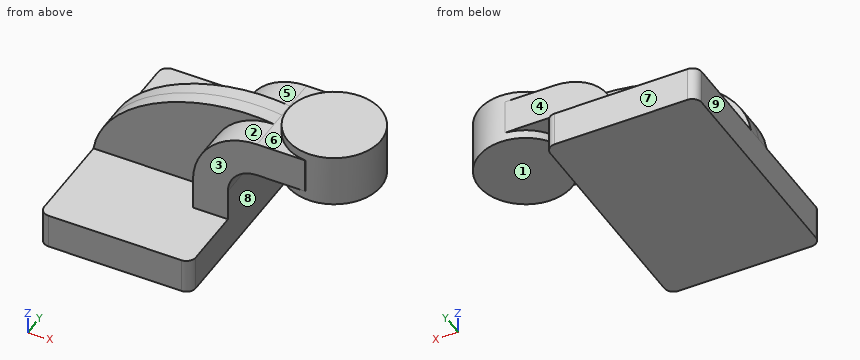
from build123d import *

# Parameters (mm, degrees)
F1_DEPTH = 63.5
F0_W     = 23.0290793641
F0_H     = 19.05
F2_DEPTH = 25.4
F3_DEPTH = 7.9375
F5_R     = 5.08


with BuildPart() as f1:
    # F0 (on Front) → F1 (new body, symmetric)
    with BuildSketch(Plane.XZ):
        Polygon((-41.275, 9.525), (-41.275, -9.525), (41.275, -9.525), (41.275, 9.525), (22.225, 9.525), align=None)
    extrude(amount=F1_DEPTH, both=True)

    # F0 (on Front) → F2 (join, symmetric)
    with BuildSketch(Plane.XZ):
        with Locations((71.839539682, 52.4002)):
            Rectangle(F0_W, F0_H)
        with BuildLine():
            Line((22.225, 9.525), (41.275, 9.525))
            Line((41.275, 9.525), (41.275, 27.0002))
            ThreePointArc((41.275, 27.0002), (45.9246798487, 38.2255201513), (57.15, 42.8752))
            Line((57.15, 42.8752), (60.325, 42.8752))
            Line((60.325, 42.8752), (60.325, 61.9252))
            Line((60.325, 61.9252), (57.15, 61.9252))
            ThreePointArc((57.15, 61.9252), (32.4542956671, 51.6959043329), (22.225, 27.0002))
            Line((22.225, 27.0002), (22.225, 9.525))
        make_face()
    extrude(amount=F2_DEPTH, both=True)

    # F0 (on Front) → F3 (join, symmetric)
    with BuildSketch(Plane.XZ):
        with BuildLine():
            add(Edge.make_bspline(
                [(-41.275, 9.525), (-36.1126549542, 44.8696576059), (15.9992650151, 68.1667476892), (57.15, 61.9252)],
                knots=[0, 0, 0, 0, 111.5045361635, 111.5045361635, 111.5045361635, 111.5045361635], degree=3))
            Line((-41.275, 9.525), (22.225, 9.525))
            Line((22.225, 9.525), (22.225, 27.0002))
            ThreePointArc((22.225, 27.0002), (32.4542956671, 51.6959043329), (57.15, 61.9252))
        make_face()
    extrude(amount=F3_DEPTH, both=True)

    # F0 (on Front) → F4 (revolve)
    with BuildSketch(Plane.XZ):
        Polygon((111.125, 66.675), (85.725, 66.675), (85.725, 52.3875), (85.725, 38.1), (111.125, 38.1), align=None)
    revolve(axis=Axis((85.725, 0, 45.24375), (0, 0, 1)))

    # F5
    f5_edges = [f1.edges().sort_by_distance(p)[0] for p in [
        (-41.275, -63.5, 0),
        (41.275, -63.5, 0),
        (41.275, 63.5, 0),
        (-41.275, 63.5, 0),
    ]]
    fillet(f5_edges, radius=F5_R)


solid = f1.part
Geometry check sheet. Reference: the model listing, model coordinates, mm. Face numbers are marked on the shaded views. A direction names the side the tool comes from. Coordinates: 2 decimals unless noted, no trailing zeros. Order: outer loops, then holes, each group sorted by start corner. A loop starts at its lowest first (then second) coordinate and runs counter-clockwise, first axis right, second up. Notation, with made-up numbers: (-5.75, -25.75) - (27.25, -25.75) arc R15 ccw to (27.25, -19.75) - close; hole circle Ø10 at (-8.5, 79). An arc over 180 degrees is marked (long way). Answer in a Markdown table with one row per item. Add a question column.
1) Cross-section at B-B, the plane x = 70. Record the cut outline in (y, z) (3 decimals).
2) Material ranges on line 1 along Y through (x, z) = (16, 42.5); line 2 along Z through (x, y) = (13, -24.5) (3 decimals); line 3 along Y through (x, z) = (77, 57), recorded low to high. Write a range as [from, to].
3) Cross-section at C-C, the plane y = -43. Record the cut outline in (x, z) (3 decimals).
4) Set-up check for the marked faces 1, 2, 3, 4 and 5: record each of +Z, -Z, +X, -X, +Y, -Y from which the full face is reachable in a straight line by a thin tool's end or side.
5) Gauge pin test, flat ends, axial feed: P1, Ø15.5, axis at x = 52, z = 32.5, coming from the -Y side; P2, Ø6, axis at x = 13, y = -21, coming from the +Z side (3 decimals); P3, Ø5, axis at y = 11, z = 17, coming from the +X side (3 decimals); P4, Ø19, axis at y = 19, z = 22.5, coming from the -X side (3 decimals). Record the tip position at first contact, or that the pin passes through.
6) Cross-section at A-A, the plane y = -20.5. Record the cut outline in (x, z) (3 decimals).
7) Release check for a two-part mould opening along X. For the marked faces 6, 7, 8 and 9 record: +X half, -X half, draft (parallel to the pull), parting line (faces both ways), or undercut.
Check result:
| question | item | result |
|---|---|---|
| 1 | outline | (-25.4, 42.875) - (-19.947, 42.875) - (-19.947, 38.1) - (19.947, 38.1) - (19.947, 42.875) - (25.4, 42.875) - (25.4, 61.925) - (19.947, 61.925) - (19.947, 66.675) - (-19.947, 66.675) - (-19.947, 61.925) - (-25.4, 61.925) - close |
| 2 | line 1 | y = [-7.94, 7.94] |
| 2 | line 2 | z = [-9.525, 9.525] |
| 2 | line 3 | y = [-25.4, 25.4] |
| 3 | outline | (-41.275, -9.525) - (41.275, -9.525) - (41.275, 9.525) - (-41.275, 9.525) - close |
| 4 | face 1 | -Z, +X, +Y, -Y |
| 4 | face 2 | +Z, -X, -Y |
| 4 | face 3 | +Z, +X, -X, -Y |
| 4 | face 4 | +Z, +X, -X, +Y |
| 4 | face 5 | +Z, -X, +Y |
| 5 | P1 | passes through |
| 5 | P2 | stops at z = 9.525 |
| 5 | P3 | stops at x = 41.275 |
| 5 | P4 | stops at x = 22.225 |
| 6 | outline | (-41.275, -9.525) - (41.275, -9.525) - (41.275, 27) arc R15.875 cw to (57.15, 42.875) - (70.728, 42.875) - (70.728, 38.1) - (100.722, 38.1) - (100.722, 66.675) - (70.728, 66.675) - (70.728, 61.925) - (57.15, 61.925) arc R34.925 ccw to (22.225, 27) - (22.225, 9.525) - (-41.275, 9.525) - close |
| 7 | face 6 | undercut |
| 7 | face 7 | draft |
| 7 | face 8 | +X half |
| 7 | face 9 | -X half |
